from build123d import *

# Parameters (mm, degrees)
F1_DEPTH = 28
F2_R     = 11
F2_R_2   = 2.5
F3_DEPTH = 2
F2_R_3   = 1.5
F4_DEPTH = 2
F5_DEPTH = 21


with BuildPart() as f1:
    # F0 (on Front) → F1 (new body)
    with BuildSketch(Plane.XZ):
        with BuildLine():
            Line((-16.1, -17.6), (16.1, -17.6))
            ThreePointArc((16.1, -17.6), (17.16066, -17.16066), (17.6, -16.1))
            Line((17.6, -16.1), (17.6, 16.1))
            ThreePointArc((17.6, 16.1), (17.16066, 17.16066), (16.1, 17.6))
            Line((16.1, 17.6), (-16.1, 17.6))
            ThreePointArc((-16.1, 17.6), (-17.16066, 17.16066), (-17.6, 16.1))
            Line((-17.6, 16.1), (-17.6, -16.1))
            ThreePointArc((-17.6, -16.1), (-17.16066, -17.16066), (-16.1, -17.6))
        make_face()
    extrude(amount=F1_DEPTH)

    # F2 (on face) → F3 (join)
    with BuildSketch(Plane.XZ.offset(28)):
        Circle(F2_R)
        Circle(F2_R_2, mode=Mode.SUBTRACT)
    extrude(amount=F3_DEPTH)

    # F2 (on face) → F4 (cut)
    with BuildSketch(Plane.XZ.offset(28)):
        with Locations((-13, 13)):
            Circle(F2_R_3)
        with Locations((13, 13)):
            Circle(F2_R_3)
        with Locations((13, -13)):
            Circle(F2_R_3)
        with Locations((-13, -13)):
            Circle(F2_R_3)
    extrude(amount=-F4_DEPTH, mode=Mode.SUBTRACT)

    # F2 (on face) → F5 (join)
    with BuildSketch(Plane.XZ.offset(28)):
        Circle(F2_R_2)
    extrude(amount=F5_DEPTH)


solid = f1.part
Design review of the part built by this model. Coordinates are the model's own, in mm. A direction names the side the tool comes from. Round coordinates to 2 decimals unless told otherwise and drop trailing zeros. Write each loop counter-clockwise with the first axis right and the second up, starting at its lowest first coordinate (ties: lowest second). Pieces come first, ordered by that corner, then holes. Notation, with made-up numbers: M 13,-1.75 L 64,-1.75 A31 ccw 64,25.25 Z; hole C 12.5,30.25 d5. An arc over 180 degrees is marked long. One line per item, written item: value. Start each with the question number.
1. Take a section at A-A on x = 0. State the section outline as (y, z) points, then the cut area to 3 significant figures.
2. Take a section at D-D on x = 13. State the section outline as (y, z) points.
3. Clearance check with flat-ended pins moving along their axes: P1, Ø12, axis at y = -35, z = -5.5, coming from the +X side; P2, Ø2.5, axis at x = 13.5, z = -13, coming from the -Y side; P3, Ø1.5, axis at x = -12.5, z = 13, coming from the -Y side. State where each tip first meets the part, or that it passes through.
4. Draft analysis for pull direction X (two halves, no side actions). For faces 3 (the face through (13, -26, 13)), 4 (the face through (17.6, -14, 0)), 5 (the face through (0, -49, 0)), state which applies: pulls with the +X half, pulls with the -X half, needs draft (parallel to the pull), parting line crosses it, or undercut.
5. Take a section at B-B on z = 7. State the section outline as (x, y) points.
6. For faces 1 (the face through (-2.38, -28.99, -10.74)), 2 (the face through (17.17, -13.8, 17.15)), list the 3-axis set-ups (+Z, -Z, +X, -X, +Y, -Y) from which the entire face can be reached by the end or side of a thin tool; tool diameter is ignored.
7. To check wall thickness, follow probe 1 along Z at (x, y) = (13, -26.7); probe 2 along Y at (x, z) = (-15, -13); probe 3 along Y at (x, z) = (-1.5, 7.5). State the ranges of each line that lie inside material, in increasing order. Write a range as from..to.
8. Take a section at C-C on y = -44. State the section outline as (x, z) points, then the cut area to 3 significant figures.
Computed:
1. outline: M -49,-2.5 L -30,-2.5 L -30,-11 L -28,-11 L -28,-17.6 L 0,-17.6 L 0,17.6 L -28,17.6 L -28,11 L -30,11 L -30,2.5 L -49,2.5 Z
1. area: 1,120 mm²
2. outline: M -28,-17.6 L 0,-17.6 L 0,17.6 L -28,17.6 L -28,14.5 L -26,14.5 L -26,11.5 L -28,11.5 L -28,-11.5 L -26,-11.5 L -26,-14.5 L -28,-14.5 Z
3. P1: stops at x = 10.78
3. P2: stops at y = -28
3. P3: stops at y = -26
4. face 3: undercut
4. face 4: pulls with the +X half
4. face 5: needs draft
5. outline: M -17.6,-28 L -8.49,-28 L -8.49,-30 L 8.49,-30 L 8.49,-28 L 17.6,-28 L 17.6,0 L -17.6,0 Z
6. face 1: -Y
6. face 2: +Z, +X, +Y, -Y
7. probe 1: z = -17.6..-14.5, -11.5..11.5, 14.5..17.6
7. probe 2: y = -28..0
7. probe 3: y = -30..0
8. outline: C 0,0 d5
8. area: 19.6 mm²
